```python
from build123d import *

# Parameters (mm, degrees)
BOSS_EXTRUDE1_DEPTH             = 6.35
F_9_64_0_14063_DIAMETER_HOLE1_D = 3.572002


with BuildPart() as part:
    # Sketch1 → Boss-Extrude1 (new body)
    with BuildSketch(Plane.XY):
        with BuildLine():
            Line((-6.35, 6.35), (-9.525, 6.35))
            Line((-9.525, 6.35), (-9.525, 12.25423))
            ThreePointArc((-9.525, 12.25423), (-3.175, 18.60423), (3.175, 12.25423))
            Line((3.175, 12.25423), (3.175, 6.35))
            Line((3.175, 6.35), (0, 6.35))
            Line((0, 6.35), (0, 0))
            Line((0, 0), (-6.35, 0))
            Line((-6.35, 0), (-6.35, 6.35))
        make_face()
    extrude(amount=BOSS_EXTRUDE1_DEPTH)

    # 9/64 (0.14063) Diameter Hole1 (through all)
    with Locations(Plane.XY.offset(6.35)):
        with Locations((-3.175, 11.80846)):
            Hole(F_9_64_0_14063_DIAMETER_HOLE1_D / 2)


solid = part.part
```
Could you check a few things on this model? Use its own coordinates, in mm. A direction names the side the tool comes from. Round coordinates to 2 decimals unless told otherwise and drop trailing zeros. Loops run counter-clockwise (first coordinate to the right, second up) from the corner with the lowest first, then second, coordinate; pieces in that order, holes last. Notation, with made-up numbers: (58, 56) - (101, 56) arc R19 ccw to (101, 78) - close; hole circle Ø5 at (-1.75, 66). An arc over 180 degrees is marked (long way). Answer as CSV lines item,"result".
1. I want a section at C-C on z = 1.5. List the corners of the cut face in (x, y) for me (3 decimals), then the cut area to 3 significant figures.
Filled in:
outline,"(-9.525, 6.35) - (-6.35, 6.35) - (-6.35, 0) - (0, 0) - (0, 6.35) - (3.175, 6.35) - (3.175, 12.254) arc R6.35 ccw to (-9.525, 12.254) - close; hole circle Ø3.572 at (-3.175, 11.808)"
area,"169 mm^2"
2. I want a section at B-B on y = 13. List the corners of the cut face in (x, z) for me, then the cut area to 3 significant figures.
Filled in:
outline,"(-9.48, 0) - (-4.51, 0) - (-4.51, 6.35) - (-9.48, 6.35) - close; (-1.84, 0) - (3.13, 0) - (3.13, 6.35) - (-1.84, 6.35) - close"
area,"63.2 mm^2"
3. I want a section at D-D on y = 2.25. List the corners of the cut face in (x, z) for me, then the cut area to 3 significant figures.
Filled in:
outline,"(-6.35, 0) - (0, 0) - (0, 6.35) - (-6.35, 6.35) - close"
area,"40.3 mm^2"
4. I want a section at A-A on x = -3.5. List the corners of the cut face in (y, z) for me, then the cut area to 3 significant figures.
Filled in:
outline,"(0, 0) - (10.05, 0) - (10.05, 6.35) - (0, 6.35) - close; (13.56, 0) - (18.6, 0) - (18.6, 6.35) - (13.56, 6.35) - close"
area,"95.8 mm^2"
5. On a 3-axis mill with a long thin cutter (end or side, diameter ignored), from which of +Z, -Z, +X, -X, +Y, -Y can I reach the whole of each face in a straight line? I mean faces 4 (the face through (3.175, 9, 3)), 5 (the face through (0, 3, 3)), 6 (the face through (-8, 6.35, 3)). Say none if no direction works.
Filled in:
face 4,"+Z, -Z, +X, +Y, -Y"
face 5,"+Z, -Z, +X, -Y"
face 6,"+Z, -Z, -X, -Y"
6. We'd pull the mould along X, two halves only. Please class faces 1 (the face through (2, 6.35, 3)), 2 (the face through (-3.315, 18.603, 3.131)), 3 (the face through (-1.859, 13.016, 3.131)): +X half, -X half, draft (parallel to the pull), parting line (faces both ways), or undercut.
Filled in:
face 1,"draft"
face 2,"parting line"
face 3,"undercut"
7. Please list where these lines run through material, in increasing order: line 1 along X through (y, z) = (5, 4); line 2 along Y through (x, z) = (-3.75, 4.5); line 3 along X through (y, z) = (12.25, 2.25) (3 decimals). Write a range as [from, to].
Filled in:
line 1,"x = [-6.35, 0]"
line 2,"y = [0, 10.12], [13.5, 18.58]"
line 3,"x = [-9.525, -4.906], [-1.444, 3.175]"
8. For pin 1 Ø3 at (x, z) = (-1.5, 2.5) entering from -Y; pin 2 Ø3 at (y, z) = (4.5, 2.5) entering from +X; pin 3 Ø2 at (x, z) = (-8, 2.5) entering from +Y; pin 4 Ø1 at (x, z) = (-7.5, 4) entering from -Y, each with a flat end and sliding along its axis, tell me the tip position at first contact or that it passes through.
Filled in:
pin 1,"stops at y = 0"
pin 2,"stops at x = 0"
pin 3,"stops at y = 17.32"
pin 4,"stops at y = 6.35"
